Check sheet for the modelled part. Datum: model origin and axes. Units: mm. Face numbers are marked on the shaded views. A direction names the side the tool comes from. Round coordinates to 2 decimals unless told otherwise and drop trailing zeros. Write each loop counter-clockwise with the first axis right and the second up, starting at its lowest first coordinate (ties: lowest second). Pieces come first, ordered by that corner, then holes. Notation, with made-up numbers: (81.25, 47) -> (115.25, 47) arc R19 ccw to (115.25, 57) -> close; hole circle Ø2 at (86.5, -16.75). An arc over 180 degrees is marked (long way). Use one line per item in the form item = value. Start each with the question number.
```python
from build123d import *

# Parameters (mm, degrees)
F0_W     = 2.25
F0_H     = 3.75
F1_DEPTH = 5
F2_W     = 1
F2_H     = 2.5
F3_DEPTH = 3.5


with BuildPart() as f1:
    # F0 (on Top) → F1 (new body)
    with BuildSketch(Plane.XY):
        with Locations((1.125, 1.875)):
            Rectangle(F0_W, F0_H)
        with Locations((-1.125, 1.875)):
            Rectangle(F0_W, F0_H)
        Polygon((2.25, 0), (0, 0), (-2.25, 0), (-2.25, -3.75), (0, -3.75), (2.25, -3.75), align=None)
    extrude(amount=-F1_DEPTH)

    # F2 (on face) → F3 (cut)
    with BuildSketch(Plane.XY):
        with Locations((0.5, 1.25)):
            Rectangle(F2_W, F2_H)
        with Locations((-0.5, 1.25)):
            Rectangle(F2_W, F2_H)
        Polygon((1, 0), (0, 0), (-1, 0), (-1, -2.5), (0, -2.5), (1, -2.5), align=None)
    extrude(amount=-F3_DEPTH, mode=Mode.SUBTRACT)


solid = f1.part
```
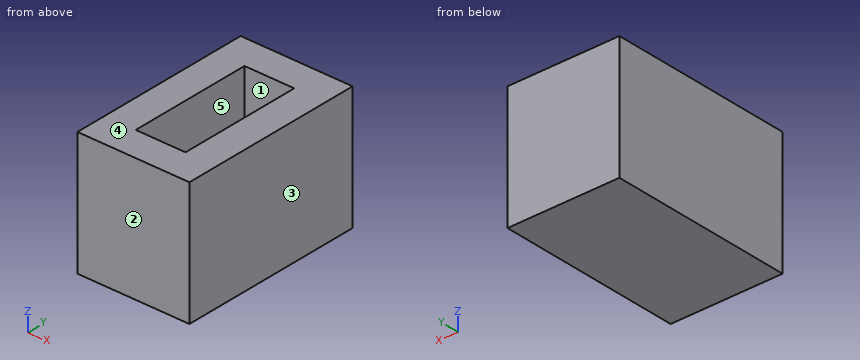
1. Sectioned sample at A-A (z = -0.4). Enter the section's corners in (x, y).
2. Scan lines: probe 1 along Y at (x, z) = (0.6, -2.6); probe 2 along X at (y, z) = (-1.75, -2.65); probe 3 along Z at (x, y) = (0.3, 0.25). Record each from-to range of solid material in increasing order.
3. Sectioned sample at C-C (x = 0.5). Enter the section's corners in (y, z), and give its area (3 significant figures).
4. Depth check by flat-ended pin: pin 1 (0.6 mm diameter, centred on x = 0.5, y = 0, fed in from +Z). Enter the tip coordinate at first touch or a pass-through.
5. Mould release check, pull along X, two halves, no side actions. Record for the marked faces 1, 2 and 3: +X half, -X half, draft (parallel to the pull), parting line (faces both ways), or undercut.
6. Tool access check on the marked faces 4 and 5. Record the directions out of +Z, -Z, +X, -X, +Y, -Y that give a thin tool (end or side, any length) a straight path to the whole face; none if there is none.
7. Sectioned sample at B-B (y = 1). Enter the section's corners in (x, z).
Returned:
q1.outline = (-2.25, -3.75) -> (2.25, -3.75) -> (2.25, 3.75) -> (-2.25, 3.75) -> close; hole (-1, -2.5) -> (1, -2.5) -> (1, 2.5) -> (-1, 2.5) -> close
q2.probe_1 = -3.75 to -2.5, 2.5 to 3.75
q2.probe_2 = -2.25 to -1, 1 to 2.25
q2.probe_3 = -5 to -3.5
q3.outline = (-3.75, -5) -> (3.75, -5) -> (3.75, 0) -> (2.5, 0) -> (2.5, -3.5) -> (-2.5, -3.5) -> (-2.5, 0) -> (-3.75, 0) -> close
q3.area = 20.0 mm^2
q4.pin_1 = -3.5
q5.face_1 = undercut
q5.face_2 = draft
q5.face_3 = +X half
q6.face_4 = +Z, +X, -X, +Y, -Y
q6.face_5 = +Z
q7.outline = (-2.25, -5) -> (2.25, -5) -> (2.25, 0) -> (1, 0) -> (1, -3.5) -> (-1, -3.5) -> (-1, 0) -> (-2.25, 0) -> close
